Read the model definition and answer for the solid it produces. Units are mm, in the model's axes. Face numbers are marked on the shaded views. A direction names the side the tool comes from. Round coordinates to 2 decimals unless told otherwise and drop trailing zeros. Order: outer loops, then holes, each group sorted by start corner. A loop starts at its lowest first (then second) coordinate and runs counter-clockwise, first axis right, second up. Notation, with made-up numbers: M -27.5,34 L -15.5,34 A6 cw -15.5,42 Z; hole C 61,-34 d3. An arc over 180 degrees is marked long. Answer as CSV lines item,"result".
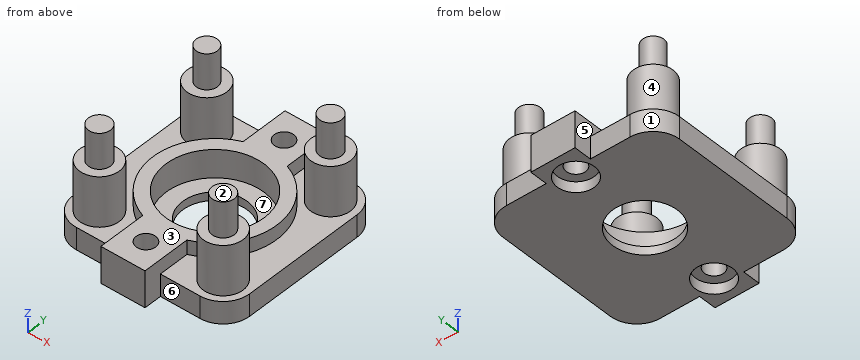
```python
from build123d import *

# Parameters (mm, degrees)
EXTRUDE_1_DEPTH     = 1.5
SKETCH_4_R          = 2.25
EXTRUDE_2_DEPTH     = 6.6
SKETCH_5_R          = 1.2
SKETCH_5_R_2        = 1.25
EXTRUDE_3_DEPTH     = 4
SKETCH_6_R          = 7
EXTRUDE_4_DEPTH     = 2.6
SKETCH_7_R          = 5.535
CUT_EXTRUDE_1_DEPTH = 3.15
SKETCH_8_R          = 3.65
CUT_EXTRUDE_2_DEPTH = 5.65
EXTRUDE_6_REACH     = 18.248
SKETCH_11_W         = 5
SKETCH_11_H         = 5.997078986
SKETCH_12_R         = 2.1
CUT_EXTRUDE_5_DEPTH = 1.2
SKETCH_13_R         = 1.1
CUT_EXTRUDE_6_DEPTH = 26.5
EXTRUDE_7_DEPTH     = 1


with BuildPart() as part:
    # 草图1 → 凸台-拉伸1 (new body)
    with BuildSketch(Plane.XY):
        with BuildLine():
            Line((-7, -10), (7, -10))
            ThreePointArc((7, -10), (9.121320344, -9.121320344), (10, -7))
            Line((10, -7), (10, 7))
            ThreePointArc((10, 7), (9.121320344, 9.121320344), (7, 10))
            Line((7, 10), (-7, 10))
            ThreePointArc((-7, 10), (-9.121320344, 9.121320344), (-10, 7))
            Line((-10, 7), (-10, -7))
            ThreePointArc((-10, -7), (-9.121320344, -9.121320344), (-7, -10))
        make_face()
    extrude(amount=EXTRUDE_1_DEPTH)

    # 草图4 → 凸台-拉伸2 (add)
    with BuildSketch(Plane.XY.offset(1.5)):
        with Locations((-7, -7)):
            Circle(SKETCH_4_R)
        with Locations((7, -7)):
            Circle(SKETCH_4_R)
        with Locations((7, 7)):
            Circle(SKETCH_4_R)
        with Locations((-7, 7)):
            Circle(SKETCH_4_R)
    extrude(amount=EXTRUDE_2_DEPTH)

    # 草图5 → 凸台-拉伸3 (add)
    with BuildSketch(Plane.XY.offset(8.1)):
        with Locations((-7, 7)):
            Circle(SKETCH_5_R)
        with Locations((-7, -7)):
            Circle(SKETCH_5_R_2)
        with Locations((7, -7)):
            Circle(SKETCH_5_R_2)
        with Locations((7, 7)):
            Circle(SKETCH_5_R_2)
    extrude(amount=EXTRUDE_3_DEPTH)

    # 草图6 → 凸台-拉伸4 (add)
    with BuildSketch(Plane.XY.offset(1.5)):
        Circle(SKETCH_6_R)
    extrude(amount=EXTRUDE_4_DEPTH)

    # 草图7 → 切除-拉伸1 (cut)
    with BuildSketch(Plane.XY.offset(4.1)):
        Circle(SKETCH_7_R)
    extrude(amount=-CUT_EXTRUDE_1_DEPTH, mode=Mode.SUBTRACT)

    # 草图8 → 切除-拉伸2 (cut)
    with BuildSketch(Plane.XY.offset(0.95)):
        Circle(SKETCH_8_R)
    extrude(amount=-CUT_EXTRUDE_2_DEPTH, mode=Mode.SUBTRACT)

    # 凸台-拉伸6: up to this face of the body (flat: up to its plane)
    extrude_6_end = Plane(part.part.faces().sort_by_distance((0, -9.717157288, 0))[0])
    # 草图11 → 凸台-拉伸6 (add, up to the picked face)
    with BuildSketch(Plane.XY.offset(4.1), mode=Mode.PRIVATE) as extrude_6_sk1:
        with Locations((0, 9.001460507)):
            Rectangle(SKETCH_11_W, SKETCH_11_H)
    extrude_6_tool1 = split(extrude(extrude_6_sk1.sketch, amount=-EXTRUDE_6_REACH, mode=Mode.PRIVATE), bisect_by=extrude_6_end, keep=Keep.BOTH, mode=Mode.PRIVATE)
    extrude_6 = extrude_6_tool1.solids().sort_by(Axis((0, 9.001461, 4.1), (0, 0, -1)))[0]
    add(extrude_6)

    # 草图12 → 切除-拉伸5 (cut)
    with BuildSketch(Plane(origin=(0, 0, 0), x_dir=(-1, 0, 0), z_dir=(0, 0, -1))):
        with Locations((0, 9)):
            Circle(SKETCH_12_R)
    cut_extrude_5 = extrude(amount=-CUT_EXTRUDE_5_DEPTH, mode=Mode.SUBTRACT)

    # 镜向1: 凸台-拉伸6, 切除-拉伸5 across plane
    add(extrude_6.mirror(Plane.ZX))
    add(cut_extrude_5.mirror(Plane.ZX), mode=Mode.SUBTRACT)

    # 草图13 → 切除-拉伸6 (cut)
    with BuildSketch(Plane(origin=(0, 0, 1.2), x_dir=(-1, 0, 0), z_dir=(0, 0, -1))):
        with Locations((0, 9)):
            Circle(SKETCH_13_R)
        with Locations((0, -9)):
            Circle(SKETCH_13_R)
    extrude(amount=-CUT_EXTRUDE_6_DEPTH, mode=Mode.SUBTRACT)

    # 草图14 → 凸台-拉伸7 (add)
    with BuildSketch(Plane.XY.offset(1.5)):
        with BuildLine():
            Line((-7, -10), (-2.5, -10))
            Line((-2.5, -10), (-2.5, -6.538348415))
            ThreePointArc((-2.5, -6.538348415), (-7, 0), (-2.5, 6.538348415))
            Line((-2.5, 6.538348415), (-2.5, 10))
            Line((-2.5, 10), (-7, 10))
            ThreePointArc((-7, 10), (-9.121320344, 9.121320344), (-10, 7))
            Line((-10, 7), (-10, -7))
            ThreePointArc((-10, -7), (-9.121320344, -9.121320344), (-7, -10))
        make_face()
        with BuildLine():
            Line((2.5, -6.538348415), (2.5, -10))
            Line((2.5, -10), (7, -10))
            ThreePointArc((7, -10), (9.121320344, -9.121320344), (10, -7))
            Line((10, -7), (10, 7))
            ThreePointArc((10, 7), (9.121320344, 9.121320344), (7, 10))
            Line((7, 10), (2.5, 10))
            Line((2.5, 10), (2.5, 6.538348415))
            ThreePointArc((2.5, 6.538348415), (7, 0), (2.5, -6.538348415))
        make_face()
    extrude(amount=EXTRUDE_7_DEPTH)


solid = part.part
```
Item 1: A cutting plane is placed at C-C, the plane y = -1. Determine the outline of the cut face in (x, z).
Ans:
outline,"M -10,0 L -3.51,0 L -3.51,0.95 L -5.44,0.95 L -5.44,4.1 L -6.93,4.1 L -6.93,2.5 L -10,2.5 Z; M 3.51,0 L 10,0 L 10,2.5 L 6.93,2.5 L 6.93,4.1 L 5.44,4.1 L 5.44,0.95 L 3.51,0.95 Z"
Item 2: A cutting plane is placed at B-B, the plane x = 0. Determine the outline of the cut face in (y, z) (3 decimals), and give its area (3 significant figures).
Ans:
outline,"M -12,0 L -11.1,0 L -11.1,1.2 L -10.1,1.2 L -10.1,4.1 L -12,4.1 Z; M -7.9,1.2 L -6.9,1.2 L -6.9,0 L -3.65,0 L -3.65,0.95 L -5.535,0.95 L -5.535,4.1 L -7.9,4.1 Z; M 3.65,0 L 6.9,0 L 6.9,1.2 L 7.9,1.2 L 7.9,4.1 L 5.535,4.1 L 5.535,0.95 L 3.65,0.95 Z; M 10.1,1.2 L 11.1,1.2 L 11.1,0 L 12,0 L 12,4.1 L 10.1,4.1 Z"
area,"33.8 mm2"
Item 3: A cutting plane is placed at D-D, the plane x = -3.25. Determine the outline of the cut face in (y, z).
Ans:
outline,"M -10,0 L -1.66,0 L -1.66,0.95 L -4.48,0.95 L -4.48,4.1 L -6.2,4.1 L -6.2,2.5 L -10,2.5 Z; M 1.66,0 L 10,0 L 10,2.5 L 6.2,2.5 L 6.2,4.1 L 4.48,4.1 L 4.48,0.95 L 1.66,0.95 Z"
Item 4: A tool of negligible diameter and unlimited length cuts with its end or side. For the marked faces 5, 6 and 7, from which of +Z, -Z, +X, -X, +Y, -Y can it reach the whole face along a straight path? Write none if from no direction.
Ans:
face 5,"+Z, +Y"
face 6,"+Z, -Z, +X, -Y"
face 7,"+Z"
Item 5: Flat-ended cylindrical pins translate along their axes: pin 1 (4 mm diameter, centred on x = 0, y = -9, fed in from +Z); pin 2 (9 mm diameter, centred on x = 0, y = 1, fed in from +Z); pin 3 (1 mm diameter, centred on x = -7, y = 9, fed in from +Z). Find the tip coordinate at first contact, or state that the pin passes through.
Ans:
pin 1,"z = 4.1"
pin 2,"z = 0.95"
pin 3,"z = 8.1"
Item 6: Determine the mould class of the marked faces 1, 2, 3 and 4 for opening direction Y: +Y half, -Y half, draft (parallel to the pull), parting line (faces both ways), or undercut.
Ans:
face 1,"+Y half"
face 2,"draft"
face 3,"undercut"
face 4,"undercut"
Item 7: Find the intervals of material crossed by probe 1 along Y at (x, z) = (0, 0.25); probe 2 along Y at (x, z) = (0, 3.2) (3 decimals); probe 3 along Z at (x, y) = (3, -5.75), in increasing order. Write a range as [from, to].
Ans:
probe 1,"[-12, -11.1], [-6.9, -3.65], [3.65, 6.9], [11.1, 12]"
probe 2,"[-12, -10.1], [-7.9, -5.535], [5.535, 7.9], [10.1, 12]"
probe 3,"[0, 4.1]"
Item 8: A cutting plane is placed at A-A, the plane z = 3. Determine the outline of the cut face in (x, y) (3 decimals).
Ans:
outline,"C -7,-7 d4.5; C -7,7 d4.5; M -2.5,-12 L 2.5,-12 L 2.5,-6.538 A7 ccw 2.5,6.538 L 2.5,12 L -2.5,12 L -2.5,6.538 A7 ccw -2.5,-6.538 Z; C 7,-7 d4.5; C 7,7 d4.5; hole C 0,0 d11.07; hole C 0,-9 d2.2; hole C 0,9 d2.2"
